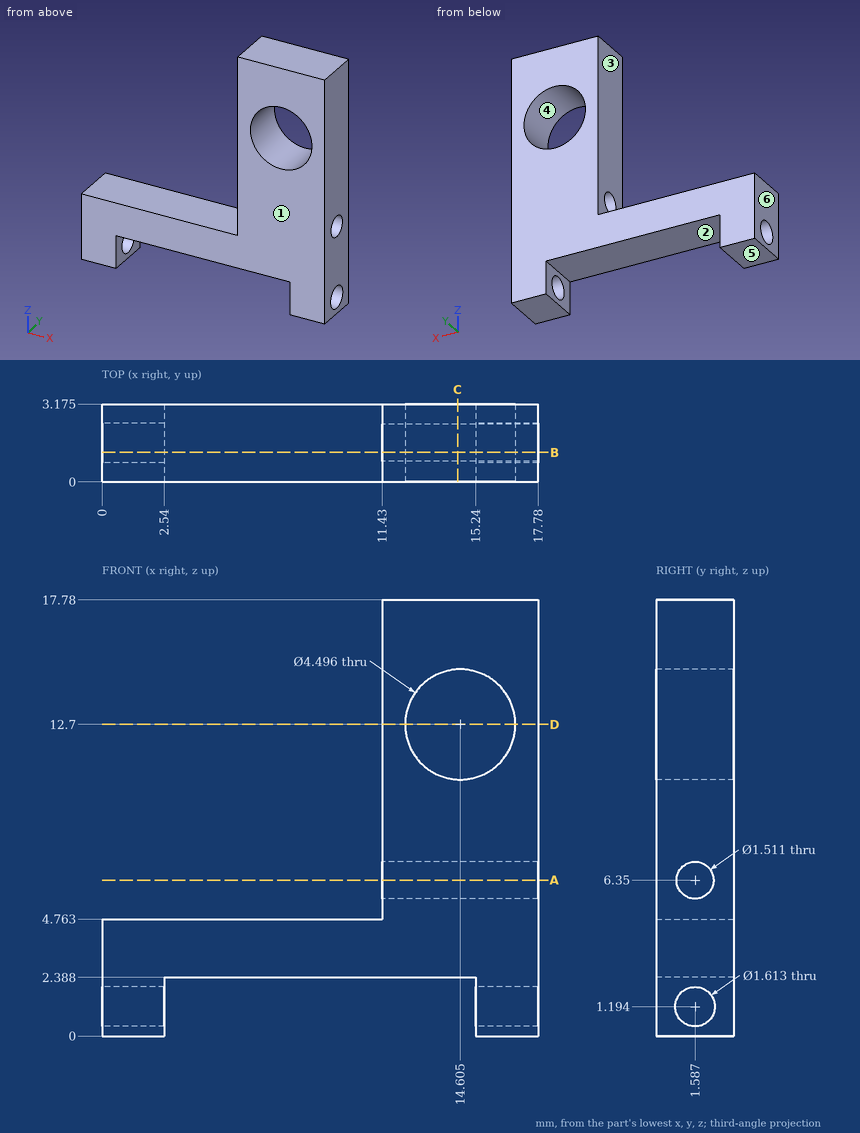
Input: dimensioned drawing with shaded views. Units: mm. Origin: part minimum x, y, z. A direction names the side the tool comes from. Give positions to 0.01 mm unless a question says otherwise; leave off trailing zeros. Write each loop counter-clockwise with the first axis right and the second up, starting at its lowest first coordinate (ties: lowest second). Pieces come first, ordered by that corner, then holes. Notation, with made-up numbers: (74, 88.5) -> (105, 88.5) arc R22 ccw to (105, 100.5) -> close; hole circle Ø3 at (-21, 69.5). An arc over 180 degrees is marked (long way). Return JSON: item names as keys, results as strings. Group by question number.
1. Section D-D, the plane z = 12.7. Output: boundary loops of the cut face in (x, y) (1 decimal).
2. Section B-B, the plane y = 1.2. Output: boundary loops of the cut face in (x, z) (1 decimal), then the cut area to 3 significant figures.
3. Mould query, pull axis X, two halves, no side actions, for the marked faces 4, 5 and 6. Classes: +X half, -X half, draft (parallel to the pull), parting line (faces both ways), or undercut.
4. Section A-A, the plane z = 6.35. Output: boundary loops of the cut face in (x, y) (1 decimal).
5. Access query for the marked faces 1, 2 and 3. Directions: +Z, -Z, +X, -X, +Y, -Y. A direction counts if a zero-diameter tool reaches every point of the face in a straight line with its end or side. Return the directions, or none.
6. Section C-C, the plane x = 14.5. Count the separate pieces of the cut face and the enclosed holes in it.
7. Material intervals for line 1 (Z direction, x = 17.25, y = 2.15) (1 decimal); line 2 (X direction, y = 3, z = 2.25); line 3 (X direction, y = 0.8, z = 10), sorted ascending. Write a range as from..to.
8. Pin query (flat end, axial travel): pin 1 Ø1 at (x, y) = (8.5, 1.5) entering from -Z. Return the tip coordinate at first contact, or that it passes through.
Determined:
{
 "1": {"outline": "(11.4, 0) -> (12.4, 0) -> (12.4, 3.2) -> (11.4, 3.2) -> close; (16.9, 0) -> (17.8, 0) -> (17.8, 3.2) -> (16.9, 3.2) -> close"},
 "2": {"outline": "(0, 0) -> (2.5, 0) -> (2.5, 0.5) -> (0, 0.5) -> close; (0, 1.9) -> (2.5, 1.9) -> (2.5, 2.4) -> (15.2, 2.4) -> (15.2, 1.9) -> (17.8, 1.9) -> (17.8, 5.7) -> (11.4, 5.7) -> (11.4, 4.8) -> (0, 4.8) -> close; (11.4, 7) -> (17.8, 7) -> (17.8, 17.8) -> (11.4, 17.8) -> close; (15.2, 0) -> (17.8, 0) -> (17.8, 0.5) -> (15.2, 0.5) -> close; hole circle Ø4.5 at (14.6, 12.7)", "area": "106 mm2"},
 "3": {"face 4": "undercut", "face 5": "draft", "face 6": "-X half"},
 "4": {"outline": "(11.4, 0) -> (17.8, 0) -> (17.8, 0.8) -> (11.4, 0.8) -> close; (11.4, 2.3) -> (17.8, 2.3) -> (17.8, 3.2) -> (11.4, 3.2) -> close"},
 "5": {"face 1": "+Z, -Z, +X, -X, -Y", "face 2": "-Z, +Y, -Y", "face 3": "+Z, -X, +Y, -Y"},
 "6": {"separate pieces": "2", "enclosed holes": "1"},
 "7": {"line 1": "z = 0..0.6, 1.8..5.8, 6.9..17.8", "line 2": "x = 0..2.54, 15.24..17.78", "line 3": "x = 11.43..17.78"},
 "8": {"pin 1": "stops at z = 2.39"}
}
